from build123d import *

# Parameters (mm, degrees)
SKETCH087_W      = 36
SKETCH087_H      = 40
SKETCH087_R      = 4.25
PAD039_DEPTH     = 24.3
FILLET015_R      = 15
POCKET045_DEPTH  = 6
CHAMFER040_SIZE  = 1
SKETCH089_W      = 16
SKETCH089_H      = 15
PAD040_DEPTH     = 6
CHAMFER041_SIZE2 = 4
CHAMFER041_SIZE  = 12
SKETCH090_R      = 2.75
POCKET046_DEPTH  = 40
SKETCH091_R      = 5.5
POCKET047_DEPTH  = 11
CHAMFER042_SIZE  = 1
CHAMFER043_SIZE  = 2
CHAMFER044_SIZE  = 0.4


with BuildPart() as obj1:
    # Sketch087 → Pad039 (new body)
    with BuildSketch(Plane.XZ):
        with Locations((-3, -5)):
            Rectangle(SKETCH087_W, SKETCH087_H)
        Circle(SKETCH087_R, mode=Mode.SUBTRACT)
    extrude(amount=-PAD039_DEPTH)

    # Fillet015
    fillet015_edges = [obj1.edges().sort_by_distance(p)[0] for p in [
        (15, 12.15, 15),
    ]]
    fillet(fillet015_edges, radius=FILLET015_R)

    # Sketch088 (on Face2 of Fillet015) → Pocket045 (cut)
    with BuildSketch(Plane.XZ):
        Polygon((7.621024, 0), (3.810512, 6.6), (-3.810512, 6.6), (-7.621024, 0), (-3.810512, -6.6), (3.810512, -6.6), align=None)
    extrude(amount=-POCKET045_DEPTH, mode=Mode.SUBTRACT)

    # Chamfer040
    chamfer040_edges = [obj1.edges().sort_by_distance(p)[0] for p in [
        (-4.25, 6, 0),
    ]]
    chamfer(chamfer040_edges, length=CHAMFER040_SIZE)

    # Sketch089 (on Face16 of Chamfer040) → Pad040 (join)
    with BuildSketch(Plane.XZ):
        with Locations((7, -17.5)):
            Rectangle(SKETCH089_W, SKETCH089_H)
    extrude(amount=PAD040_DEPTH)

    # Chamfer041
    chamfer041_edges = [obj1.edges().sort_by_distance(p)[0] for p in [
        (15, -6, -17.5),
    ]]
    chamfer041_side = obj1.faces().sort_by_distance((7, -6, -17.5))[0]
    chamfer(chamfer041_edges, length=CHAMFER041_SIZE, length2=CHAMFER041_SIZE2, reference=chamfer041_side)

    # Sketch090 (on Face9 of Chamfer041) → Pocket046 (cut)
    with BuildSketch(Plane(origin=(0, 24.3, 0), x_dir=(-1, 0, 0), z_dir=(0, 1, 0))):
        with Locations((11, -17)):
            Circle(SKETCH090_R)
    extrude(amount=-POCKET046_DEPTH, mode=Mode.SUBTRACT)

    # Sketch091 (on Face9 of Pocket046) → Pocket047 (cut)
    with BuildSketch(Plane(origin=(0, 24.3, 0), x_dir=(-1, 0, 0), z_dir=(0, 1, 0))):
        with Locations((11, -17)):
            Circle(SKETCH091_R)
    extrude(amount=-POCKET047_DEPTH, mode=Mode.SUBTRACT)

    # Chamfer042
    chamfer042_edges = [obj1.edges().sort_by_distance(p)[0] for p in [
        (-5.5, 24.3, -17),
        (-4.25, 24.3, 0),
        (-8.25, 13.3, -17),
    ]]
    chamfer(chamfer042_edges, length=CHAMFER042_SIZE)

    # Chamfer043
    chamfer043_edges = [obj1.edges().sort_by_distance(p)[0] for p in [
        (-21, 0, -5),
        (-21, 24.3, -5),
        (-10.5, 24.3, 15),
        (15, 0, -5),
    ]]
    chamfer(chamfer043_edges, length=CHAMFER043_SIZE)

    # Chamfer044
    chamfer044_edges = [obj1.edges().sort_by_distance(p)[0] for p in [
        (15, 10.15, -25),
        (14, 23.3, -25),
        (9, -4, -25),
        (-3, 24.3, -25),
        (1, -6, -25),
        (-20, 23.3, -25),
        (-1, -3, -25),
        (-21, 12.15, -25),
        (-10, 0, -25),
        (-20, 1, -25),
    ]]
    chamfer(chamfer044_edges, length=CHAMFER044_SIZE)


with BuildPart() as obj1_1:
    # Body024 placement: moved
    add(obj1.part.moved(Location((0, -70, 0))))


with BuildPart() as part_mirroring004:
    # Part__Mirroring004: instance of obj1
    add(obj1_1.part.mirror(Plane(origin=(0, 0, 0), x_dir=(1, 0, 0), z_dir=(0, 1, 0))))


solid = part_mirroring004.part
Model file for the job. Use its own axes, mm. A direction names the side the tool comes from. Coordinates: 2 decimals unless noted, no trailing zeros. Loops run counter-clockwise (first coordinate to the right, second up) from the corner with the lowest first, then second, coordinate; pieces in that order, holes last. Notation, with made-up numbers: (87, -27.75) -> (119, -27.75) arc R24 cw to (119, -1.75) -> close; hole circle Ø7 at (73, 65.25). An arc over 180 degrees is marked (long way). Use one line per item in the form item = value. Start each with the question number.
(1) Cut at C-C on y = 62.5. Give the cut face in (x, z), and give its area (3 significant figures).
(2) Pull direction Z, two halves, no side cores. Call faces 6 (the flat face through (15, 60, -12)), 7 (the flat face through (5.742, 67.042, 3.254)), 8 (the flat face through (5, 72, -10)): pulls with the +Z half, pulls with the -Z half, needs draft (parallel to the pull), parting line crosses it, or undercut.
(3) Flat gauge pins, fed straight in: pin 1 (10 mm diameter, centred on x = -15, z = 0, fed in from +Y); pin 2 (2.5 mm diameter, centred on x = 6.5, y = 71, fed in from +Z); pin 3 (5 mm diameter, centred on y = 73, z = -20, fed in from -X). Where does each tip first touch, or does it go through?
(4) Tool access for faces 1 (the flat face through (-10, 69, 14)), 2 (the flat face through (-20, 46.7, -5.1)), 3 (the flat face through (0, 67, -6.6)), 4 (the flat face through (14, 69, -5)), 5 (the flat face through (-15, 56.7, -18)): list every direction of +Z, -Z, +X, -X, +Y, -Y with a clear straight run to the whole face (end or side of a thin tool).
(5) Cut at B-B on y = 53.5. Give the cut face in (x, z), and give its area (3 significant figures).
(6) Probe probe 1 along Z at (x, y) = (-11, 54); probe 2 along Z at (x, y) = (-11, 67); probe 3 along Y at (x, z) = (-13.5, 2). List the from-to ranges inside material, lowest first. Write a range as from..to.
(7) Cut at A-A on x = -11. Give the cut face in (y, z), and give its area (3 significant figures).
Values:
q1.outline = (-21, -24.6) -> (-20.6, -25) -> (14.6, -25) -> (15, -24.6) -> (15, 0) arc R15 ccw to (0, 15) -> (-21, 15) -> close; hole circle Ø5.5 at (-11, -17); hole circle Ø8.5 at (0, 0)
q1.area = 1,310 mm2
q2.face_6 = needs draft
q2.face_7 = undercut
q2.face_8 = pulls with the +Z half
q3.pin_1 = 70
q3.pin_2 = 11.7
q3.pin_3 = -1
q4.face_1 = +Z, +X, -X, +Y
q4.face_2 = +Z, -Z, -X, -Y
q4.face_3 = +Y
q4.face_4 = +Z, +X, +Y
q4.face_5 = -Y
q5.outline = (-21, -24.6) -> (-20.6, -25) -> (14.6, -25) -> (15, -24.6) -> (15, 0) arc R15 ccw to (0, 15) -> (-21, 15) -> close; hole circle Ø11 at (-11, -17); hole circle Ø8.5 at (0, 0)
q5.area = 1,240 mm2
q6.probe_1 = -25..-22.5, -11.5..15
q6.probe_2 = -25..-19.75, -14.25..15
q6.probe_3 = 45.7..70
q7.outline = (45.7, -24.6) -> (46.1, -25) -> (69.6, -25) -> (70, -24.6) -> (70, -19.75) -> (57.7, -19.75) -> (56.7, -20.75) -> (56.7, -22.5) -> (46.7, -22.5) -> (45.7, -23.5) -> close; (45.7, -10.5) -> (46.7, -11.5) -> (56.7, -11.5) -> (56.7, -13.25) -> (57.7, -14.25) -> (70, -14.25) -> (70, 13) -> (68, 15) -> (47.7, 15) -> (45.7, 13) -> close
q7.area = 772 mm2
